```python
from build123d import *

# Parameters (mm, degrees)
SKETCH1_R           = 5
BOSS_EXTRUDE1_DEPTH = 18.5
BOSS_EXTRUDE2_DEPTH = 10
SKETCH4_W           = 5.25
SKETCH4_H           = 5.25
CUT_EXTRUDE2_DEPTH  = 10


with BuildPart() as part:
    # Sketch1 → Boss-Extrude1 (new body)
    with BuildSketch(Plane.XY):
        Circle(SKETCH1_R)
    extrude(amount=BOSS_EXTRUDE1_DEPTH)

    # Sketch3 → Boss-Extrude2 (add)
    with BuildSketch(Plane.XY.offset(18.5)):
        with BuildLine():
            ThreePointArc((-4, -3), (-3.535533906, -3.535533906), (-3, -4))
            Line((-3, -4), (3, -4))
            ThreePointArc((3, -4), (3.535533906, -3.535533906), (4, -3))
            Line((4, -3), (4, 3))
            ThreePointArc((4, 3), (3.535533906, 3.535533906), (3, 4))
            Line((3, 4), (-3, 4))
            ThreePointArc((-3, 4), (-3.535533906, 3.535533906), (-4, 3))
            Line((-4, 3), (-4, -3))
        make_face()
    extrude(amount=BOSS_EXTRUDE2_DEPTH)

    # Sketch4 → Cut-Extrude2 (cut)
    with BuildSketch(Plane.XY.offset(28.5)):
        Rectangle(SKETCH4_W, SKETCH4_H)
    extrude(amount=-CUT_EXTRUDE2_DEPTH, mode=Mode.SUBTRACT)


solid = part.part
```
Check sheet for the modelled part. Datum: model origin and axes. Units: mm. A direction names the side the tool comes from. Coordinates: 2 decimals unless noted, no trailing zeros. Loops run counter-clockwise (first coordinate to the right, second up) from the corner with the lowest first, then second, coordinate; pieces in that order, holes last.
1) Material ranges on probe 1 along X at (y, z) = (0, 18.75) (3 decimals); probe 2 along X at (y, z) = (-4, 3.25), recorded low to high.
2) Sectioned sample at B-B (z = 22). Record the boundary of the cut face in (x, y) (3 decimals).
3) Access from +Z, -Z, +X, -X, +Y, -Y to the whole of each face (thin tool, end or side, straight path). Record for faces 4 (the face through (0, 4.4, 18.5)), 5 (the face through (-4.4, 0, 18.5)), 6 (the face through (0, 2.625, 24)).
4) Gauge pin test, flat ends, axial feed: pin 1 (3 mm diameter, centred on x = 0, z = 24.5, fed in from +Y); pin 2 (1.6 mm diameter, centred on x = 1, y = 0, fed in from +Z); pin 3 (2.5 mm diameter, centred on y = -1, z = 23, fed in from -X). Record the tip position at first contact, or that the pin passes through.
5) Release check for a two-part mould opening along Y. For faces 1 (the face through (2.625, 0, 24)), 2 (the face through (0, -4, 23)), 3 (the face through (4, 0, 23)) record: released by +Y, released by -Y, zero draft, split by the parting line, or undercut.
6) Sectioned sample at A-A (y = 0). Record the boundary of the cut face in (x, z) (3 decimals), and give its area (4 significant figures).
7) Sectioned sample at D-D (z = 16.75). Record the boundary of the cut face in (x, y).
Check sheet entries:
1. probe 1: x = -4 to -2.625, 2.625 to 4
1. probe 2: x = -3 to 3
2. outline: (-4, -3) arc R5 ccw to (-3, -4) - (3, -4) arc R5 ccw to (4, -3) - (4, 3) arc R5 ccw to (3, 4) - (-3, 4) arc R5 ccw to (-4, 3) - close; hole (-2.625, -2.625) - (2.625, -2.625) - (2.625, 2.625) - (-2.625, 2.625) - close
3. face 4: +Z, +X, -X, +Y
3. face 5: +Z, -X, +Y, -Y
3. face 6: +Z
4. pin 1: stops at y = 4
4. pin 2: stops at z = 18.5
4. pin 3: stops at x = -4
5. face 1: undercut
5. face 2: released by -Y
5. face 3: zero draft
6. outline: (-5, 0) - (5, 0) - (5, 18.5) - (4, 18.5) - (4, 28.5) - (2.625, 28.5) - (2.625, 18.5) - (-2.625, 18.5) - (-2.625, 28.5) - (-4, 28.5) - (-4, 18.5) - (-5, 18.5) - close
6. area: 212.5 mm2
7. outline: circle Ø10 at (0, 0)
